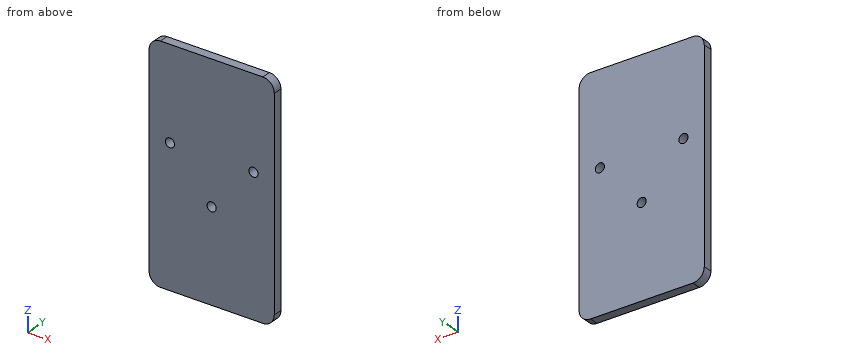
```python
from build123d import *

# Parameters (mm, degrees)
SKETCH1_R           = 1
BOSS_EXTRUDE1_DEPTH = 2


with BuildPart() as part:
    # Sketch1 → Boss-Extrude1 (new body)
    with BuildSketch(Plane(origin=(0, 0, 0), x_dir=(1, 0, 0), z_dir=(0, 1, 0))):
        with BuildLine():
            Line((-11.25, -25), (11.25, -25))
            ThreePointArc((11.25, -25), (13.017766953, -24.267766953), (13.75, -22.5))
            Line((13.75, -22.5), (13.75, 22.5))
            ThreePointArc((13.75, 22.5), (13.017766953, 24.267766953), (11.25, 25))
            Line((11.25, 25), (-11.25, 25))
            ThreePointArc((-11.25, 25), (-13.017766953, 24.267766953), (-13.75, 22.5))
            Line((-13.75, 22.5), (-13.75, -22.5))
            ThreePointArc((-13.75, -22.5), (-13.017766953, -24.267766953), (-11.25, -25))
        make_face()
        with Locations((0, 5)):
            Circle(SKETCH1_R, mode=Mode.SUBTRACT)
        with Locations((-9.18, -5)):
            Circle(SKETCH1_R, mode=Mode.SUBTRACT)
        with Locations((9.18, -5)):
            Circle(SKETCH1_R, mode=Mode.SUBTRACT)
    extrude(amount=BOSS_EXTRUDE1_DEPTH)


solid = part.part
```
For this review, take the finished solid that the model builds, in its own axes (mm). Give positions to 0.01 mm unless a question says otherwise; leave off trailing zeros. Write each loop counter-clockwise with the first axis right and the second up, starting at its lowest first coordinate (ties: lowest second). Pieces come first, ordered by that corner, then holes.
Item 1: Take a section at A-A (z = -5). Give the boundary of the cut face in (x, y).
Item 2: Take a section at B-B (x = 9.18). Give the boundary of the cut face in (y, z), and give its area (3 significant figures).
Item 3: Wall thickness on probe 1 along X at (y, z) = (1.3, 5); probe 2 along Z at (x, y) = (9.18, 0.5); probe 3 along Z at (x, y) = (0, 1.3): over which ranges is each line inside the solid? List them lowest first.
Established:
1. outline: (-13.75, 0) - (-1, 0) - (-1, 2) - (-13.75, 2) - close; (1, 0) - (13.75, 0) - (13.75, 2) - (1, 2) - close
2. outline: (0, -25) - (2, -25) - (2, 4) - (0, 4) - close; (0, 6) - (2, 6) - (2, 25) - (0, 25) - close
2. area: 96.0 mm2
3. probe 1: x = -13.75 to -10.18, -8.18 to 8.18, 10.18 to 13.75
3. probe 2: z = -25 to 4, 6 to 25
3. probe 3: z = -25 to -6, -4 to 25
